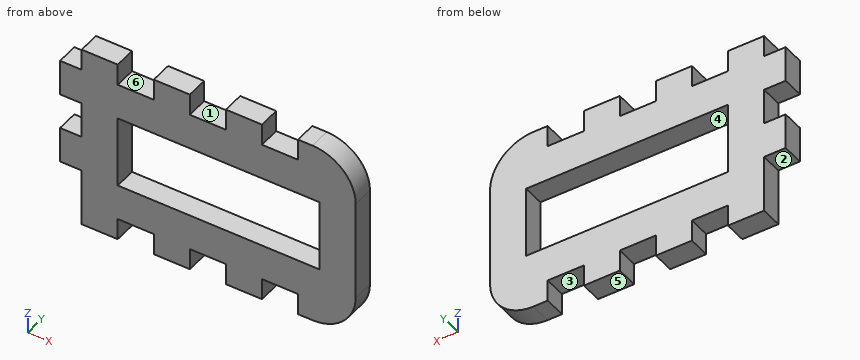
from build123d import *

# Parameters (mm, degrees)
SKETCH1_W           = 38
SKETCH1_H           = 26
BOSS_EXTRUDE1_DEPTH = 1.5
SKETCH8_W           = 5
SKETCH8_H           = 3
BOSS_EXTRUDE2_DEPTH = 3
SKETCH9_W           = 5
SKETCH9_H           = 3
CUT_EXTRUDE2_DEPTH  = 3
FILLET1_R           = 6
SKETCH10_W          = 28
SKETCH10_H          = 10
CUT_EXTRUDE3_DEPTH  = 3


with BuildPart() as part:
    # Sketch1 → Boss-Extrude1 (new body, symmetric)
    with BuildSketch(Plane(origin=(0, 0, 0), x_dir=(1, 0, 0), z_dir=(0, 1, 0))):
        Rectangle(SKETCH1_W, SKETCH1_H)
    extrude(amount=BOSS_EXTRUDE1_DEPTH, both=True)

    # Sketch8 → Boss-Extrude2 (add)
    with BuildSketch(Plane.ZY.offset(19)):
        with Locations((-2.5, 0)):
            Rectangle(SKETCH8_W, SKETCH8_H)
        with Locations((7.5, 0)):
            Rectangle(SKETCH8_W, SKETCH8_H)
    extrude(amount=BOSS_EXTRUDE2_DEPTH)

    # Sketch9 → Cut-Extrude2 (cut)
    with BuildSketch(Plane.XZ.offset(1.5)):
        with Locations((-11.5, -11.5)):
            Rectangle(SKETCH9_W, SKETCH9_H)
        with Locations((-11.5, 11.5)):
            Rectangle(SKETCH9_W, SKETCH9_H)
        with Locations((-1.5, -11.5)):
            Rectangle(SKETCH9_W, SKETCH9_H)
        with Locations((-1.5, 11.5)):
            Rectangle(SKETCH9_W, SKETCH9_H)
        with Locations((8.5, -11.5)):
            Rectangle(SKETCH9_W, SKETCH9_H)
        with Locations((8.5, 11.5)):
            Rectangle(SKETCH9_W, SKETCH9_H)
    extrude(amount=-CUT_EXTRUDE2_DEPTH, mode=Mode.SUBTRACT)

    # Fillet1
    fillet1_edges = [part.edges().sort_by_distance(p)[0] for p in [
        (19, 0, 13),
        (19, 0, -13),
    ]]
    fillet(fillet1_edges, radius=FILLET1_R)

    # Sketch10 → Cut-Extrude3 (cut)
    with BuildSketch(Plane(origin=(0, 1.5, 0), x_dir=(1, 0, 0), z_dir=(0, 1, 0))):
        Rectangle(SKETCH10_W, SKETCH10_H)
    extrude(amount=-CUT_EXTRUDE3_DEPTH, mode=Mode.SUBTRACT)


solid = part.part
Can you work these out from the model? Positions are in its coordinate system, mm. Face numbers are marked on the shaded views. A direction names the side the tool comes from. Coordinates: 2 decimals unless noted, no trailing zeros. Write each loop counter-clockwise with the first axis right and the second up, starting at its lowest first coordinate (ties: lowest second). Pieces come first, ordered by that corner, then holes. Notation, with made-up numbers: (82.25, 15) -> (132.25, 15) arc R15 ccw to (132.25, 31) -> close; hole circle Ø3 at (-34.75, -34). An arc over 180 degrees is marked (long way). Write item = value, one per line.
(1) On a 3-axis mill with a long thin cutter (end or side, diameter ignored), from which of +Z, -Z, +X, -X, +Y, -Y can I reach the whole of each face in a straight line? I mean the marked faces 1, 2 and 3. Say none if no direction works.
Verdict:
face_1 = +Z, +Y, -Y
face_2 = -Z, -X, +Y, -Y
face_3 = -Z, +Y, -Y
(2) If I drill on probe 1 along Z at (x, y) = (-2.5, 0.7); probe 2 along Z at (x, y) = (13, -0.05); probe 3 along X at (y, z) = (0.5, 12), over which ranges is the centre line in solid material (lowest first)?
Verdict:
probe_1 = -10 to -5, 5 to 10
probe_2 = -13 to -5, 5 to 13
probe_3 = -19 to -14, -9 to -4, 1 to 6, 11 to 16.32
(3) Imagine slicing it at D-D (x = 15.5). Please give me the cut outline in (y, z).
Verdict:
outline = (-1.5, -12.45) -> (1.5, -12.45) -> (1.5, 12.45) -> (-1.5, 12.45) -> close
(4) Thinking about a two-plate mould opening in Z: for the marked faces 4, 5 and 6, which applies, +Z half, -Z half, draft (parallel to the pull), parting line (faces both ways), or undercut?
Verdict:
face_4 = undercut
face_5 = -Z half
face_6 = +Z half
(5) Imagine slicing it at B-B (z = 2.5). Please give me the cut outline in (x, y).
Verdict:
outline = (-19, -1.5) -> (-14, -1.5) -> (-14, 1.5) -> (-19, 1.5) -> close; (14, -1.5) -> (19, -1.5) -> (19, 1.5) -> (14, 1.5) -> close
(6) Imagine slicing it at A-A (x = -11.5). Please give me the cut outline in (y, z).
Verdict:
outline = (-1.5, -10) -> (1.5, -10) -> (1.5, -5) -> (-1.5, -5) -> close; (-1.5, 5) -> (1.5, 5) -> (1.5, 10) -> (-1.5, 10) -> close
(7) For pin 1 (0.9 mm diameter, centred on y = 0, z = -11, fed in from -X); pin 2 (1.5 mm diameter, centred on y = 0, z = 12, fed in from +X); pin 3 (1.5 mm diameter, centred on y = 0.5, z = -11.5, fed in from +X), each with a flat end and sliding along its axis, tell me the tip position at first contact or that it passes through.
Verdict:
pin_1 = -19
pin_2 = 17.24
pin_3 = 17.68
(8) Imagine slicing it at C-C (z = -11.5). Please give me the cut outline in (x, y).
Verdict:
outline = (-19, -1.5) -> (-14, -1.5) -> (-14, 1.5) -> (-19, 1.5) -> close; (-9, -1.5) -> (-4, -1.5) -> (-4, 1.5) -> (-9, 1.5) -> close; (1, -1.5) -> (6, -1.5) -> (6, 1.5) -> (1, 1.5) -> close; (11, -1.5) -> (16.97, -1.5) -> (16.97, 1.5) -> (11, 1.5) -> close
